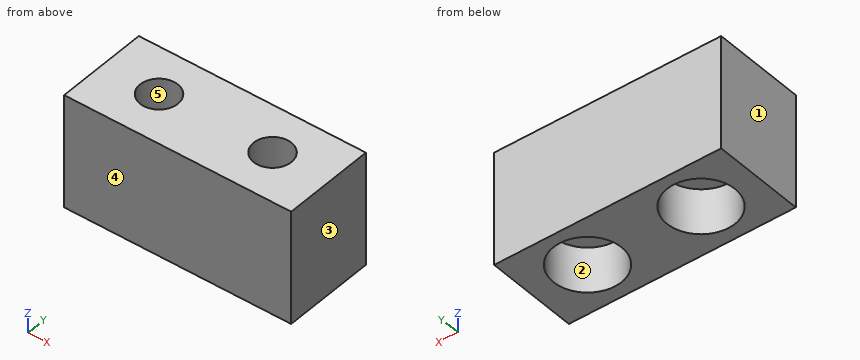
from build123d import *

# Parameters (mm, degrees)
SKETCH1_W           = 30
SKETCH1_H           = 14.7
SKETCH1_R           = 2.5
BOSS_EXTRUDE1_DEPTH = 15
SKETCH4_R           = 4.5
CUT_EXTRUDE1_DEPTH  = 6
SKETCH6_W           = 43.790019277
SKETCH6_H           = 8.282134106
CUT_EXTRUDE2_DEPTH  = 23.45044543


with BuildPart() as part:
    # Sketch1 → Boss-Extrude1 (new body)
    with BuildSketch(Plane.XY):
        Rectangle(SKETCH1_W, SKETCH1_H)
        with Locations((7.5, 1.35)):
            Circle(SKETCH1_R, mode=Mode.SUBTRACT)
        with Locations((-7.5, 1.35)):
            Circle(SKETCH1_R, mode=Mode.SUBTRACT)
    extrude(amount=BOSS_EXTRUDE1_DEPTH)

    # Sketch4 → Cut-Extrude1 (cut)
    with BuildSketch(Plane(origin=(0, 0, 0), x_dir=(-1, 0, 0), z_dir=(0, 0, -1))):
        with Locations((-7.5, 1.35)):
            Circle(SKETCH4_R)
        with Locations((7.5, 1.35)):
            Circle(SKETCH4_R)
    extrude(amount=-CUT_EXTRUDE1_DEPTH, mode=Mode.SUBTRACT)

    # Sketch6 → Cut-Extrude2 (cut, through all)
    with BuildSketch(Plane(origin=(0, 0, 0), x_dir=(-1, 0, 0), z_dir=(0, 0, -1))):
        with Locations((2.714530428, -9.041067053)):
            Rectangle(SKETCH6_W, SKETCH6_H)
    extrude(amount=-CUT_EXTRUDE2_DEPTH, mode=Mode.SUBTRACT)


solid = part.part
Can you work these out from the model? Positions are in its coordinate system, mm. Face numbers are marked on the shaded views. A direction names the side the tool comes from. Round coordinates to 2 decimals unless told otherwise and drop trailing zeros. Write each loop counter-clockwise with the first axis right and the second up, starting at its lowest first coordinate (ties: lowest second). Pieces come first, ordered by that corner, then holes. Notation, with made-up numbers: (-20, 44.5) -> (-14, 44.5) arc R23 cw to (-14, 54.5) -> close; hole circle Ø1 at (50.25, 40.5). An arc over 180 degrees is marked (long way). Use one line per item in the form item = value. Start each with the question number.
Q1. Which directions (+Z, -Z, +X, -X, +Y, -Y) give clear straight access to the entire face, cutting with the end or side of a thin tool? Please do the marked faces 1 and 2.
Q2. Imagine slicing it at D-D (x = 8). Please give me the cut outline in (y, z), then the cut area to 3 significant figures.
Q3. Imagine slicing it at A-A (x = -7.5). Please give me the cut outline in (y, z), then the cut area to 4 significant figures.
Q4. I'm going to push a flat-ended pin straight in: P1, Ø2.5, axis at x = -9.5, y = 3.5, coming from the -Z side. Where does the tip first touch, or does it pass through?
Q5. Imagine slicing it at C-C (z = 10.75). Please give me the cut outline in (x, y).
Q6. Imagine slicing it at B-B (y = 1.35). Please give me the cut outline in (x, z).
Q7. We'd pull the mould along Y, two halves only. Please class the marked faces 3, 4 and 5: +Y half, -Y half, draft (parallel to the pull), parting line (faces both ways), or undercut.
Q8. If I drill on probe 1 along X at (y, z) = (1.35, 12.75); probe 2 along Y at (x, z) = (-7.5, 2.2); probe 3 along Y at (x, z) = (-7.5, 13), over which ranges is the centre line in solid material (lowest first)? Write a range as [from, to].
Worked out:
q1.face_1 = +Z, -Z, -X, +Y, -Y
q1.face_2 = -Z
q2.outline = (-4.9, 0) -> (-3.12, 0) -> (-3.12, 6) -> (-1.1, 6) -> (-1.1, 15) -> (-4.9, 15) -> close; (3.8, 6) -> (5.82, 6) -> (5.82, 0) -> (7.35, 0) -> (7.35, 15) -> (3.8, 15) -> close
q2.area = 86.0 mm^2
q3.outline = (-4.9, 0) -> (-3.15, 0) -> (-3.15, 6) -> (-1.15, 6) -> (-1.15, 15) -> (-4.9, 15) -> close; (3.85, 6) -> (5.85, 6) -> (5.85, 0) -> (7.35, 0) -> (7.35, 15) -> (3.85, 15) -> close
q3.area = 84.75 mm^2
q4.P1 = 6
q5.outline = (-15, -4.9) -> (15, -4.9) -> (15, 7.35) -> (-15, 7.35) -> close; hole circle Ø5 at (-7.5, 1.35); hole circle Ø5 at (7.5, 1.35)
q6.outline = (-15, 0) -> (-12, 0) -> (-12, 6) -> (-10, 6) -> (-10, 15) -> (-15, 15) -> close; (-5, 6) -> (-3, 6) -> (-3, 0) -> (3, 0) -> (3, 6) -> (5, 6) -> (5, 15) -> (-5, 15) -> close; (10, 6) -> (12, 6) -> (12, 0) -> (15, 0) -> (15, 15) -> (10, 15) -> close
q7.face_3 = draft
q7.face_4 = -Y half
q7.face_5 = undercut
q8.probe_1 = [-15, -10], [-5, 5], [10, 15]
q8.probe_2 = [-4.9, -3.15], [5.85, 7.35]
q8.probe_3 = [-4.9, -1.15], [3.85, 7.35]
